Work out the finished part from the listing and answer in its coordinate system (mm). Face numbers are marked on the shaded views. A direction names the side the tool comes from. Round coordinates to 2 decimals unless told otherwise and drop trailing zeros. Order: outer loops, then holes, each group sorted by start corner. A loop starts at its lowest first (then second) coordinate and runs counter-clockwise, first axis right, second up. Notation, with made-up numbers: (43, 22) -> (86, 22) arc R27 ccw to (86, 54) -> close; hole circle Ø11 at (-23.5, 70). An arc over 180 degrees is marked (long way). Use a Markdown table: item, result. Add a question column.
Item 1: A tool of negligible diameter and unlimited length cuts with its end or side. For the marked faces 1 and 2, from which of +Z, -Z, +X, -X, +Y, -Y can it reach the whole face along a straight path? Write none if from no direction.
Item 2: A cutting plane is placed at D-D, the plane x = 1. Determine the outline of the cut face in (y, z), plus the area to 3 significant figures.
Item 3: A cutting plane is placed at A-A, the plane x = -5.75. Determine the outline of the cut face in (y, z), plus the area to 3 significant figures.
Item 4: A cutting plane is placed at C-C, the plane y = 1.2. Determine the outline of the cut face in (x, z).
Item 5: Flat-ended cylindrical pins translate along their axes: P1, Ø1.8, axis at y = 3.5, z = 5.5, coming from the -X side; P2, Ø1.1, axis at x = -1, z = -6, coming from the -Y side; P3, Ø1.5, axis at x = -9.5, z = -4, coming from the +Y side; P4, Ø1.3, axis at y = 3, z = 4.5, coming from the +X side. Find the tip coordinate at first contact, or state that the pin passes through.
Item 6: Find the intervals of material crossed by L1, parallel to Z at x = 0, y = 3.6; L2, parallel to X at y = 3, z = 6.75; L3, parallel to X at y = 3.65, z = -6.5, in increasing order. Write a range as [from, to].
Item 7: A cutting plane is placed at B-B, the plane z = -4.75. Determine the outline of the cut face in (x, y), plus the area to 3 significant figures.
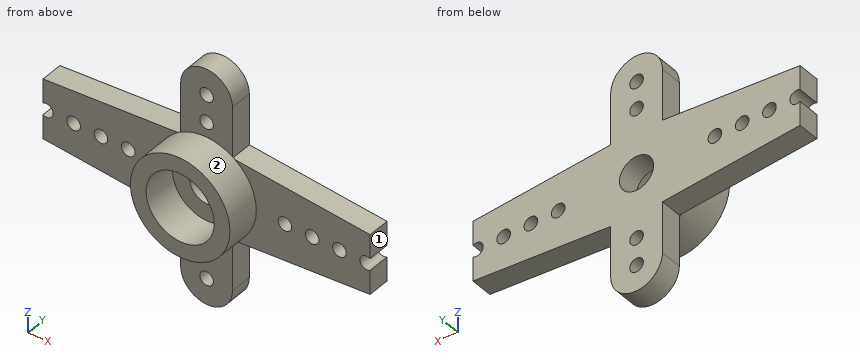
from build123d import *

# Parameters (mm, degrees)
SKETCH1_R           = 3.65
SKETCH1_R_2         = 2.5
BOSS_EXTRUDE1_DEPTH = 2.5
SKETCH2_R           = 1.25
BOSS_EXTRUDE2_DEPTH = 1.6
CUT_EXTRUDE1_REACH  = 6.1
SKETCH3_R           = 0.5
SKETCH4_W           = 8.285333373
SKETCH4_H           = 11.992925475
CUT_EXTRUDE2_DEPTH  = 5.1


with BuildPart() as part:
    # Sketch1 → Boss-Extrude1 (new body)
    with BuildSketch(Plane(origin=(0, 0, 0), x_dir=(1, 0, 0), z_dir=(0, 1, 0))):
        Circle(SKETCH1_R)
        Circle(SKETCH1_R_2, mode=Mode.SUBTRACT)
    extrude(amount=BOSS_EXTRUDE1_DEPTH)

    # Sketch2 → Boss-Extrude2 (add)
    with BuildSketch(Plane(origin=(0, 2.5, 0), x_dir=(1, 0, 0), z_dir=(0, 1, 0))):
        with BuildLine():
            Line((-1.9, 6.75), (-1.9, 3))
            Line((-1.9, 3), (-15.75, 1.9))
            ThreePointArc((-15.75, 1.9), (-17.65, 0), (-15.75, -1.9))
            Line((-15.75, -1.9), (-1.9, -3))
            Line((-1.9, -3), (-1.9, -6.75))
            ThreePointArc((-1.9, -6.75), (0, -8.65), (1.9, -6.75))
            Line((1.9, -6.75), (1.9, -3))
            Line((1.9, -3), (15.75, -1.9))
            ThreePointArc((15.75, -1.9), (17.65, 0), (15.75, 1.9))
            Line((15.75, 1.9), (1.9, 3))
            Line((1.9, 3), (1.9, 6.75))
            ThreePointArc((1.9, 6.75), (0, 8.65), (-1.9, 6.75))
        make_face()
        Circle(SKETCH2_R, mode=Mode.SUBTRACT)
    extrude(amount=BOSS_EXTRUDE2_DEPTH)

    # Sketch3 → Cut-Extrude1 (cut, up to next)
    with BuildSketch(Plane(origin=(0, 4.1, 0), x_dir=(1, 0, 0), z_dir=(0, 1, 0)), mode=Mode.PRIVATE) as cut_extrude1_sk1:
        with Locations((0, 6.75)):
            Circle(SKETCH3_R)
    cut_extrude1_tool1 = extrude(cut_extrude1_sk1.sketch, amount=-CUT_EXTRUDE1_REACH, mode=Mode.PRIVATE) & part.part
    add(cut_extrude1_tool1.solids().sort_by_distance((0, 4.1, -6.75))[0], mode=Mode.SUBTRACT)
    # Sketch3 → Cut-Extrude1 (cut, up to next)
    with BuildSketch(Plane(origin=(0, 4.1, 0), x_dir=(1, 0, 0), z_dir=(0, 1, 0)), mode=Mode.PRIVATE) as cut_extrude1_sk2:
        with Locations((0, 4.75)):
            Circle(SKETCH3_R)
    cut_extrude1_tool2 = extrude(cut_extrude1_sk2.sketch, amount=-CUT_EXTRUDE1_REACH, mode=Mode.PRIVATE) & part.part
    add(cut_extrude1_tool2.solids().sort_by_distance((0, 4.1, -4.75))[0], mode=Mode.SUBTRACT)
    # Sketch3 → Cut-Extrude1 (cut, up to next)
    with BuildSketch(Plane(origin=(0, 4.1, 0), x_dir=(1, 0, 0), z_dir=(0, 1, 0)), mode=Mode.PRIVATE) as cut_extrude1_sk3:
        with Locations((-15.75, 0)):
            Circle(SKETCH3_R)
    cut_extrude1_tool3 = extrude(cut_extrude1_sk3.sketch, amount=-CUT_EXTRUDE1_REACH, mode=Mode.PRIVATE) & part.part
    add(cut_extrude1_tool3.solids().sort_by_distance((-15.75, 4.1, 0))[0], mode=Mode.SUBTRACT)
    # Sketch3 → Cut-Extrude1 (cut, up to next)
    with BuildSketch(Plane(origin=(0, 4.1, 0), x_dir=(1, 0, 0), z_dir=(0, 1, 0)), mode=Mode.PRIVATE) as cut_extrude1_sk4:
        with Locations((-13.75, 0)):
            Circle(SKETCH3_R)
    cut_extrude1_tool4 = extrude(cut_extrude1_sk4.sketch, amount=-CUT_EXTRUDE1_REACH, mode=Mode.PRIVATE) & part.part
    add(cut_extrude1_tool4.solids().sort_by_distance((-13.75, 4.1, 0))[0], mode=Mode.SUBTRACT)
    # Sketch3 → Cut-Extrude1 (cut, up to next)
    with BuildSketch(Plane(origin=(0, 4.1, 0), x_dir=(1, 0, 0), z_dir=(0, 1, 0)), mode=Mode.PRIVATE) as cut_extrude1_sk5:
        with Locations((-11.75, 0)):
            Circle(SKETCH3_R)
    cut_extrude1_tool5 = extrude(cut_extrude1_sk5.sketch, amount=-CUT_EXTRUDE1_REACH, mode=Mode.PRIVATE) & part.part
    add(cut_extrude1_tool5.solids().sort_by_distance((-11.75, 4.1, 0))[0], mode=Mode.SUBTRACT)
    # Sketch3 → Cut-Extrude1 (cut, up to next)
    with BuildSketch(Plane(origin=(0, 4.1, 0), x_dir=(1, 0, 0), z_dir=(0, 1, 0)), mode=Mode.PRIVATE) as cut_extrude1_sk6:
        with Locations((-9.75, 0)):
            Circle(SKETCH3_R)
    cut_extrude1_tool6 = extrude(cut_extrude1_sk6.sketch, amount=-CUT_EXTRUDE1_REACH, mode=Mode.PRIVATE) & part.part
    add(cut_extrude1_tool6.solids().sort_by_distance((-9.75, 4.1, 0))[0], mode=Mode.SUBTRACT)
    # Sketch3 → Cut-Extrude1 (cut, up to next)
    with BuildSketch(Plane(origin=(0, 4.1, 0), x_dir=(1, 0, 0), z_dir=(0, 1, 0)), mode=Mode.PRIVATE) as cut_extrude1_sk7:
        with Locations((-7.75, 0)):
            Circle(SKETCH3_R)
    cut_extrude1_tool7 = extrude(cut_extrude1_sk7.sketch, amount=-CUT_EXTRUDE1_REACH, mode=Mode.PRIVATE) & part.part
    add(cut_extrude1_tool7.solids().sort_by_distance((-7.75, 4.1, 0))[0], mode=Mode.SUBTRACT)
    # Sketch3 → Cut-Extrude1 (cut, up to next)
    with BuildSketch(Plane(origin=(0, 4.1, 0), x_dir=(1, 0, 0), z_dir=(0, 1, 0)), mode=Mode.PRIVATE) as cut_extrude1_sk8:
        with Locations((-5.75, 0)):
            Circle(SKETCH3_R)
    cut_extrude1_tool8 = extrude(cut_extrude1_sk8.sketch, amount=-CUT_EXTRUDE1_REACH, mode=Mode.PRIVATE) & part.part
    add(cut_extrude1_tool8.solids().sort_by_distance((-5.75, 4.1, 0))[0], mode=Mode.SUBTRACT)
    # Sketch3 → Cut-Extrude1 (cut, up to next)
    with BuildSketch(Plane(origin=(0, 4.1, 0), x_dir=(1, 0, 0), z_dir=(0, 1, 0)), mode=Mode.PRIVATE) as cut_extrude1_sk9:
        with Locations((5.75, 0)):
            Circle(SKETCH3_R)
    cut_extrude1_tool9 = extrude(cut_extrude1_sk9.sketch, amount=-CUT_EXTRUDE1_REACH, mode=Mode.PRIVATE) & part.part
    add(cut_extrude1_tool9.solids().sort_by_distance((5.75, 4.1, 0))[0], mode=Mode.SUBTRACT)
    # Sketch3 → Cut-Extrude1 (cut, up to next)
    with BuildSketch(Plane(origin=(0, 4.1, 0), x_dir=(1, 0, 0), z_dir=(0, 1, 0)), mode=Mode.PRIVATE) as cut_extrude1_sk10:
        with Locations((7.75, 0)):
            Circle(SKETCH3_R)
    cut_extrude1_tool10 = extrude(cut_extrude1_sk10.sketch, amount=-CUT_EXTRUDE1_REACH, mode=Mode.PRIVATE) & part.part
    add(cut_extrude1_tool10.solids().sort_by_distance((7.75, 4.1, 0))[0], mode=Mode.SUBTRACT)
    # Sketch3 → Cut-Extrude1 (cut, up to next)
    with BuildSketch(Plane(origin=(0, 4.1, 0), x_dir=(1, 0, 0), z_dir=(0, 1, 0)), mode=Mode.PRIVATE) as cut_extrude1_sk11:
        with Locations((9.75, 0)):
            Circle(SKETCH3_R)
    cut_extrude1_tool11 = extrude(cut_extrude1_sk11.sketch, amount=-CUT_EXTRUDE1_REACH, mode=Mode.PRIVATE) & part.part
    add(cut_extrude1_tool11.solids().sort_by_distance((9.75, 4.1, 0))[0], mode=Mode.SUBTRACT)
    # Sketch3 → Cut-Extrude1 (cut, up to next)
    with BuildSketch(Plane(origin=(0, 4.1, 0), x_dir=(1, 0, 0), z_dir=(0, 1, 0)), mode=Mode.PRIVATE) as cut_extrude1_sk12:
        with Locations((11.75, 0)):
            Circle(SKETCH3_R)
    cut_extrude1_tool12 = extrude(cut_extrude1_sk12.sketch, amount=-CUT_EXTRUDE1_REACH, mode=Mode.PRIVATE) & part.part
    add(cut_extrude1_tool12.solids().sort_by_distance((11.75, 4.1, 0))[0], mode=Mode.SUBTRACT)
    # Sketch3 → Cut-Extrude1 (cut, up to next)
    with BuildSketch(Plane(origin=(0, 4.1, 0), x_dir=(1, 0, 0), z_dir=(0, 1, 0)), mode=Mode.PRIVATE) as cut_extrude1_sk13:
        with Locations((13.75, 0)):
            Circle(SKETCH3_R)
    cut_extrude1_tool13 = extrude(cut_extrude1_sk13.sketch, amount=-CUT_EXTRUDE1_REACH, mode=Mode.PRIVATE) & part.part
    add(cut_extrude1_tool13.solids().sort_by_distance((13.75, 4.1, 0))[0], mode=Mode.SUBTRACT)
    # Sketch3 → Cut-Extrude1 (cut, up to next)
    with BuildSketch(Plane(origin=(0, 4.1, 0), x_dir=(1, 0, 0), z_dir=(0, 1, 0)), mode=Mode.PRIVATE) as cut_extrude1_sk14:
        with Locations((15.75, 0)):
            Circle(SKETCH3_R)
    cut_extrude1_tool14 = extrude(cut_extrude1_sk14.sketch, amount=-CUT_EXTRUDE1_REACH, mode=Mode.PRIVATE) & part.part
    add(cut_extrude1_tool14.solids().sort_by_distance((15.75, 4.1, 0))[0], mode=Mode.SUBTRACT)
    # Sketch3 → Cut-Extrude1 (cut, up to next)
    with BuildSketch(Plane(origin=(0, 4.1, 0), x_dir=(1, 0, 0), z_dir=(0, 1, 0)), mode=Mode.PRIVATE) as cut_extrude1_sk15:
        with Locations((0, -4.75)):
            Circle(SKETCH3_R)
    cut_extrude1_tool15 = extrude(cut_extrude1_sk15.sketch, amount=-CUT_EXTRUDE1_REACH, mode=Mode.PRIVATE) & part.part
    add(cut_extrude1_tool15.solids().sort_by_distance((0, 4.1, 4.75))[0], mode=Mode.SUBTRACT)
    # Sketch3 → Cut-Extrude1 (cut, up to next)
    with BuildSketch(Plane(origin=(0, 4.1, 0), x_dir=(1, 0, 0), z_dir=(0, 1, 0)), mode=Mode.PRIVATE) as cut_extrude1_sk16:
        with Locations((0, -6.75)):
            Circle(SKETCH3_R)
    cut_extrude1_tool16 = extrude(cut_extrude1_sk16.sketch, amount=-CUT_EXTRUDE1_REACH, mode=Mode.PRIVATE) & part.part
    add(cut_extrude1_tool16.solids().sort_by_distance((0, 4.1, 6.75))[0], mode=Mode.SUBTRACT)

    # Sketch4 → Cut-Extrude2 (cut, through all)
    with BuildSketch(Plane(origin=(0, 4.1, 0), x_dir=(1, 0, 0), z_dir=(0, 1, 0))):
        with Locations((-16.142666687, 0.926898026)):
            Rectangle(SKETCH4_W, SKETCH4_H)
        with Locations((16.142666687, 0.926898026)):
            Rectangle(SKETCH4_W, SKETCH4_H)
    extrude(amount=-CUT_EXTRUDE2_DEPTH, mode=Mode.SUBTRACT)


solid = part.part
Reported:
| question | item | result |
|---|---|---|
| 1 | face 1 | +Z, -Z, +X, +Y, -Y |
| 1 | face 2 | -Y |
| 2 | outline | (0, -3.51) -> (2.5, -3.51) -> (2.5, -8.37) -> (4.1, -8.37) -> (4.1, -0.75) -> (2.5, -0.75) -> (2.5, -2.29) -> (0, -2.29) -> close; (0, 2.29) -> (2.5, 2.29) -> (2.5, 0.75) -> (4.1, 0.75) -> (4.1, 8.37) -> (2.5, 8.37) -> (2.5, 3.51) -> (0, 3.51) -> close |
| 2 | area | 30.5 mm² |
| 3 | outline | (2.5, -2.69) -> (4.1, -2.69) -> (4.1, -0.5) -> (2.5, -0.5) -> close; (2.5, 0.5) -> (4.1, 0.5) -> (4.1, 2.69) -> (2.5, 2.69) -> close |
| 3 | area | 7.02 mm² |
| 4 | outline | circle Ø7.3 at (0, 0); hole circle Ø5 at (0, 0) |
| 5 | P1 | x = -1.9 |
| 5 | P2 | y = 2.5 |
| 5 | P3 | through |
| 5 | P4 | x = 1.9 |
| 6 | L1 | [-8.65, -7.25], [-6.25, -5.25], [-4.25, -1.25], [1.25, 4.25], [5.25, 6.25], [7.25, 8.65] |
| 6 | L2 | [-1.9, -0.5], [0.5, 1.9] |
| 6 | L3 | [-1.9, -0.43], [0.43, 1.9] |
| 7 | outline | (-1.9, 2.5) -> (-0.5, 2.5) -> (-0.5, 4.1) -> (-1.9, 4.1) -> close; (0.5, 2.5) -> (1.9, 2.5) -> (1.9, 4.1) -> (0.5, 4.1) -> close |
| 7 | area | 4.48 mm² |
